from build123d import *

# Parameters (mm, degrees)
SKETCH1_R           = 25
SKETCH1_R_2         = 7.5
BOSS_EXTRUDE1_DEPTH = 2
SKETCH3_W           = 2.436097603
SKETCH3_H           = 25
BOSS_EXTRUDE2_DEPTH = 15
SKETCH3_3_W         = 2.436097603
SKETCH3_3_H         = 25
BOSS_EXTRUDE3_DEPTH = 15
CUT_EXTRUDE3_DEPTH  = 1
SKETCH10_R          = 1.2
CUT_EXTRUDE4_DEPTH  = 9


with BuildPart() as part:
    # Sketch1 → Boss-Extrude1 (new body)
    with BuildSketch(Plane(origin=(0, 0, 0), x_dir=(0, 1, 0), z_dir=(0, 0, 1))):
        with Locations(Location((0, 0, 0), (0, 0, 270))):
            Circle(SKETCH1_R)
        with Locations(Location((0, 0, 0), (0, 0, 270))):
            Circle(SKETCH1_R_2, mode=Mode.SUBTRACT)
    extrude(amount=BOSS_EXTRUDE1_DEPTH)

    # Sketch3 → Boss-Extrude2 (add)
    with BuildSketch(Plane.XY.offset(2)):
        with Locations((-20.432586294, 0)):
            Rectangle(SKETCH3_W, SKETCH3_H)
    extrude(amount=BOSS_EXTRUDE2_DEPTH)

    # Sketch3_3 → Boss-Extrude3 (add)
    with BuildSketch(Plane.XY.offset(2)):
        with Locations((20.432586294, 0)):
            Rectangle(SKETCH3_3_W, SKETCH3_3_H)
        with Locations((-20.432586294, 0)):
            Rectangle(SKETCH3_3_W, SKETCH3_3_H)
    extrude(amount=BOSS_EXTRUDE3_DEPTH)

    # Sketch9 → Cut-Extrude3 (cut)
    with BuildSketch(Plane.YZ.offset(21.650635095)):
        with BuildLine():
            Line((-7.8, 16.2), (7.9, 16.2))
            Line((7.9, 16.2), (7.9, 13))
            ThreePointArc((7.9, 13), (11.1, 9.8), (7.9, 6.6))
            Line((7.9, 6.6), (7.9, 3.4))
            Line((7.9, 3.4), (-7.8, 3.4))
            Line((-7.8, 3.4), (-7.8, 6.6))
            ThreePointArc((-7.8, 6.6), (-11, 9.8), (-7.8, 13))
            Line((-7.8, 13), (-7.8, 16.2))
        make_face()
    extrude(amount=-CUT_EXTRUDE3_DEPTH, mode=Mode.SUBTRACT)

    # Sketch10 → Cut-Extrude4 (cut)
    with BuildSketch(Plane.YZ.offset(21.650635095)):
        with Locations(Location((-0.968507973, 3.2, 0), (0, 0, 270))):
            Circle(SKETCH10_R)
    extrude(amount=-CUT_EXTRUDE4_DEPTH, mode=Mode.SUBTRACT)


solid = part.part
Part model, mm, in its own coordinate system. A direction names the side the tool comes from. Give positions to 0.01 mm unless a question says otherwise; leave off trailing zeros. Order: outer loops, then holes, each group sorted by start corner. A loop starts at its lowest first (then second) coordinate and runs counter-clockwise, first axis right, second up. Notation, with made-up numbers: (78, -34) - (108, -34) arc R14 cw to (108, -20) - close; hole circle Ø3 at (-3.75, 31.5). An arc over 180 degrees is marked (long way). Use a Markdown table: item, result.
1) Saw through at A-A on z = 9.8. List the corners of the cut face in (x, y), plus the area to 3 significant figures.
Checked values:
| item | result |
|---|---|
| outline | (-21.65, -12.5) - (-19.21, -12.5) - (-19.21, 12.5) - (-21.65, 12.5) - close; (19.21, -12.5) - (21.65, -12.5) - (21.65, -11) - (20.65, -11) - (20.65, 11.1) - (21.65, 11.1) - (21.65, 12.5) - (19.21, 12.5) - close |
| area | 99.7 mm² |
2) 3-axis set-ups, long thin cutter, end or side, ignore diameter. For faces 4 (the flat face through (20, -12.5, 9)), 5 (the flat face through (20, 12.5, 9)), 6 (the flat face through (-21.651, 0, 9)), 7 (the flat face through (21.651, -3, 3)): which of +Z, -Z, +X, -X, +Y, -Y reach the whole face in a straight line?
Checked values:
| item | result |
|---|---|
| face 4 | +Z, +X, -X, -Y |
| face 5 | +Z, +X, -X, +Y |
| face 6 | +Z, -X, +Y, -Y |
| face 7 | +Z, +X, +Y, -Y |
3) Two-plate mould, pull along Z, no slides. Class faces 1 (the cylindrical face through (21.2, 11.1, 9.9)), 2 (the flat face through (19.215, 0, 9)), 3 (the flat face through (-20, 0, 17)): +Z half, -Z half, draft (parallel to the pull), parting line (faces both ways), or undercut.
Checked values:
| item | result |
|---|---|
| face 1 | undercut |
| face 2 | draft |
| face 3 | +Z half |
4) Saw through at B-B on y = 3.5. List the corners of the cut face in (x, z), plus the area to 3 significant figures.
Checked values:
| item | result |
|---|---|
| outline | (-24.75, 0) - (-6.63, 0) - (-6.63, 2) - (-19.21, 2) - (-19.21, 17) - (-21.65, 17) - (-21.65, 2) - (-24.75, 2) - close; (6.63, 0) - (24.75, 0) - (24.75, 2) - (21.65, 2) - (21.65, 3.4) - (20.65, 3.4) - (20.65, 16.2) - (21.65, 16.2) - (21.65, 17) - (19.21, 17) - (19.21, 2) - (6.63, 2) - close |
| area | 133 mm² |
5) Saw through at D-D on x = 1. List the corners of the cut face in (y, z), plus the area to 3 significant figures.
Checked values:
| item | result |
|---|---|
| outline | (-24.98, 0) - (-7.43, 0) - (-7.43, 2) - (-24.98, 2) - close; (7.43, 0) - (24.98, 0) - (24.98, 2) - (7.43, 2) - close |
| area | 70.2 mm² |
6) Flat gauge pins, fed straight in: P1, Ø2.5, axis at x = -20.5, z = 10, coming from the +Y side; P2, Ø3, axis at x = 10, y = -17, coming from the +Z side; P3, Ø1.1, axis at x = 21, z = 5, coming from the -Y side; P4, Ø5, axis at x = 15, z = 7, coming from the -Y side. Where does each tip first touch, or does it go through?
Checked values:
| item | result |
|---|---|
| P1 | y = 12.5 |
| P2 | z = 2 |
| P3 | y = -12.5 |
| P4 | through |
7) Saw through at C-C on x = -20. List the corners of the cut face in (y, z).
Checked values:
| item | result |
|---|---|
| outline | (-15, 0) - (15, 0) - (15, 2) - (12.5, 2) - (12.5, 17) - (-12.5, 17) - (-12.5, 2) - (-15, 2) - close |
8) Probe L1, parallel to Y at x = 0, z = 0.8; L2, parallel to X at y = -3, z = 4.5; L3, parallel to Z at x = 5, y = 9.5. List the from-to ranges inside material, lowest first. Write a range as from..to.
Checked values:
| item | result |
|---|---|
| L1 | -25..-7.5, 7.5..25 |
| L2 | -21.65..-19.21, 19.21..20.65 |
| L3 | 0..2 |
